from build123d import *

# Parameters (mm, degrees)
MODEL_W                 = 3
MODEL_H                 = 3
SALIENTE_EXTRUIR1_DEPTH = 3


with BuildPart() as part:
    # Model → Saliente-Extruir1 (new body)
    with BuildSketch(Plane.XY):
        with BuildLine():
            Line((11.870836217, 297.491184957), (65.870836217, 297.491184957))
            ThreePointArc((65.870836217, 297.491184957), (70.370836217, 292.991184957), (65.870836217, 288.491184957))
            Line((65.870836217, 288.491184957), (11.870836217, 288.491184957))
            ThreePointArc((11.870836217, 288.491184957), (7.370836217, 292.991184957), (11.870836217, 297.491184957))
        make_face()
        with Locations((11.870836217, 292.991184957)):
            Rectangle(MODEL_W, MODEL_H, mode=Mode.SUBTRACT)
        with Locations((20.870836217, 292.991184957)):
            Rectangle(MODEL_W, MODEL_H, mode=Mode.SUBTRACT)
        with Locations((29.870836217, 292.991184957)):
            Rectangle(MODEL_W, MODEL_H, mode=Mode.SUBTRACT)
        with Locations((38.870836217, 292.991184957)):
            Rectangle(MODEL_W, MODEL_H, mode=Mode.SUBTRACT)
        with Locations((47.870836217, 292.991184957)):
            Rectangle(MODEL_W, MODEL_H, mode=Mode.SUBTRACT)
        with Locations((56.870836217, 292.991184957)):
            Rectangle(MODEL_W, MODEL_H, mode=Mode.SUBTRACT)
        with Locations((65.870836217, 292.991184957)):
            Rectangle(MODEL_W, MODEL_H, mode=Mode.SUBTRACT)
    extrude(amount=SALIENTE_EXTRUIR1_DEPTH)


solid = part.part
Check sheet for the modelled part. Datum: model origin and axes. Units: mm. A direction names the side the tool comes from. Give positions to 0.01 mm unless a question says otherwise; leave off trailing zeros. Loops run counter-clockwise (first coordinate to the right, second up) from the corner with the lowest first, then second, coordinate; pieces in that order, holes last. Notation, with made-up numbers: M 24.5,70 L 28.5,70 A14 ccw 28.5,95 Z; hole C 89,25 d3. An arc over 180 degrees is marked long. Use a Markdown table: item, result. Add a question column.
Q1. Tool access check on faces 5 (the flat face through (39, 288.491, 1)), 6 (the flat face through (13.371, 293, 1)). Record the directions out of +Z, -Z, +X, -X, +Y, -Y that give a thin tool (end or side, any length) a straight path to the whole face; none if there is none.
Q2. Sectioned sample at A-A, the plane y = 293. Give the number of separate pieces and of enclosed holes in the cut face, then the cut area to 3 significant figures.
Q3. Sectioned sample at D-D, the plane y = 296.25. Record the cut outline in (x, z), then the cut area to 3 significant figures.
Q4. Scan lines: line 1 along Y through (x, z) = (22, 2.6); line 2 along X through (y, z) = (289.75, 2.7); line 3 along X through (y, z) = (290, 0.55). Record each from-to range of solid material in increasing order. Write a range as [from, to].
Q5. Go/stop test with flat-tipped pins: pin 1 (1.5 mm diameter, centred on y = 293.5, z = 1.5, fed in from -X); pin 2 (1 mm diameter, centred on y = 294.5, z = 2.5, fed in from +X). Record where each tip stops, or that it passes through.
Q6. Mould release check, pull along X, two halves, no side actions. Record for faces 1 (the flat face through (57, 294.491, 1)), 2 (the flat face through (12, 291.491, 1)), 3 (the flat face through (39, 295, 3)), 4 (the cylindrical face through (7.37, 292.89, 1.48)): pulls with the +X half, pulls with the -X half, needs draft (parallel to the pull), parting line crosses it, or undercut.
Q7. Sectioned sample at B-B, the plane x = 65. Record the cut outline in (y, z), then the cut area to 3 significant figures.
Verdict:
| question | item | result |
|---|---|---|
| 1 | face 5 | +Z, -Z, +X, -X, -Y |
| 1 | face 6 | +Z, -Z |
| 2 | separate pieces | 8 |
| 2 | enclosed holes | 0 |
| 2 | area | 126 mm^2 |
| 3 | outline | M 8.77,0 L 68.97,0 L 68.97,3 L 8.77,3 Z |
| 3 | area | 181 mm^2 |
| 4 | line 1 | [288.49, 291.49], [294.49, 297.49] |
| 4 | line 2 | [8.75, 68.99] |
| 4 | line 3 | [8.51, 69.23] |
| 5 | pin 1 | x = 7.37 |
| 5 | pin 2 | x = 70.26 |
| 6 | face 1 | undercut |
| 6 | face 2 | undercut |
| 6 | face 3 | needs draft |
| 6 | face 4 | pulls with the -X half |
| 7 | outline | M 288.49,0 L 291.49,0 L 291.49,3 L 288.49,3 Z; M 294.49,0 L 297.49,0 L 297.49,3 L 294.49,3 Z |
| 7 | area | 18.0 mm^2 |
